Verification items for this drawing (mm, ordinates from the low corner). A direction names the side the tool comes from. Round coordinates to 2 decimals unless told otherwise and drop trailing zeros. Loops run counter-clockwise (first coordinate to the right, second up) from the corner with the lowest first, then second, coordinate; pieces in that order, holes last. Notation, with made-up numbers: M 44,89 L 82,89 A9 cw 82,102 Z; hole C 53,-5 d9. An arc over 180 degrees is marked long. Answer as CSV lines item,"result".
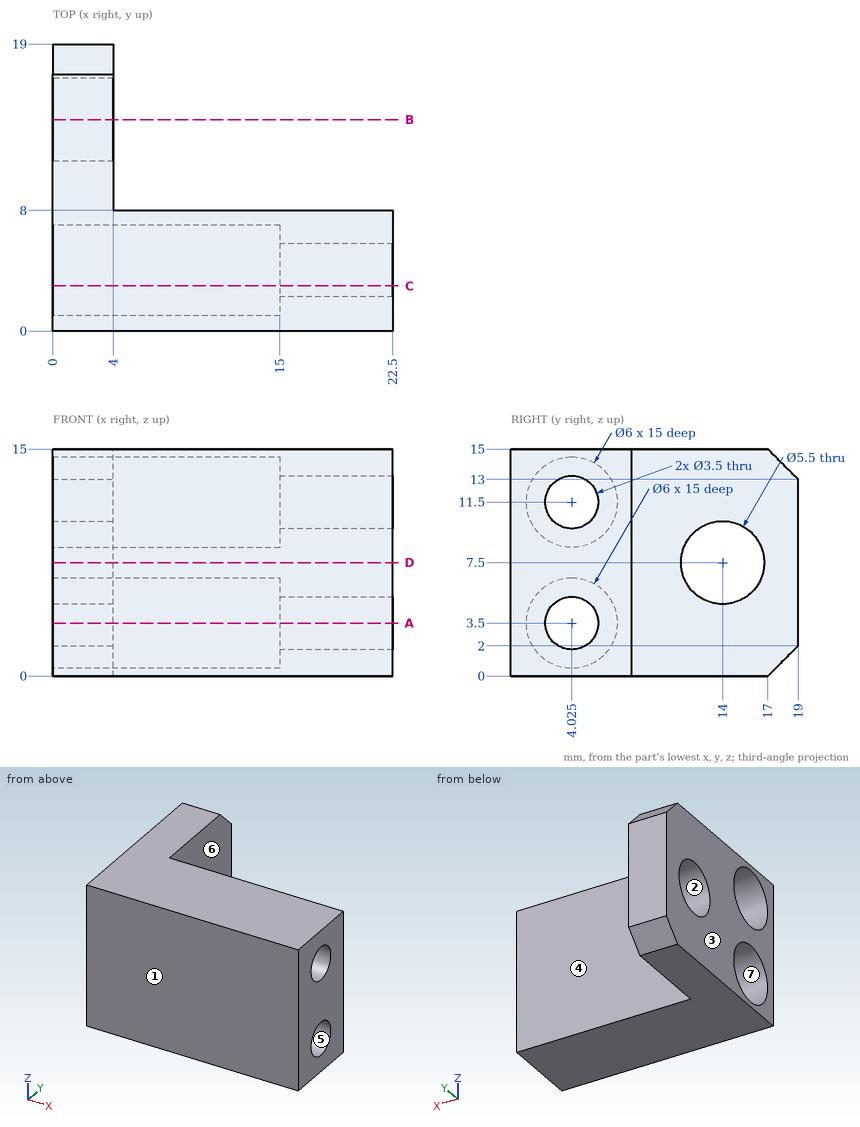
1) Section check C-C (y = 3). Record the cut outline in (x, z).
Here are the results:
outline,"M 0,0 L 22.5,0 L 22.5,2.08 L 15,2.08 L 15,0.68 L 0,0.68 Z; M 0,6.32 L 15,6.32 L 15,4.92 L 22.5,4.92 L 22.5,10.08 L 15,10.08 L 15,8.68 L 0,8.68 Z; M 0,14.32 L 15,14.32 L 15,12.92 L 22.5,12.92 L 22.5,15 L 0,15 Z"
2) Section check B-B (y = 14). Record the cut outline in (x, z), plus the area to 3 significant figures.
Here are the results:
outline,"M 0,0 L 4,0 L 4,4.75 L 0,4.75 Z; M 0,10.25 L 4,10.25 L 4,15 L 0,15 Z"
area,"38.0 mm^2"
3) Draft check along Y on the marked faces 1, 2, 3 and 4. Enter one of: +Y half, -Y half, draft (parallel to the pull), parting line (faces both ways), or undercut.
Here are the results:
face 1,"-Y half"
face 2,"undercut"
face 3,"draft"
face 4,"+Y half"
4) Section check D-D (z = 7.5). Record the cut outline in (x, y).
Here are the results:
outline,"M 0,0 L 22.5,0 L 22.5,8 L 4,8 L 4,11.25 L 0,11.25 Z; M 0,16.75 L 4,16.75 L 4,19 L 0,19 Z"
5) Section check A-A (z = 3.5). Record the cut outline in (x, y) (3 decimals), plus the area to 3 significant figures.
Here are the results:
outline,"M 0,0 L 22.5,0 L 22.5,2.275 L 15,2.275 L 15,1.025 L 0,1.025 Z; M 0,7.025 L 15,7.025 L 15,5.775 L 22.5,5.775 L 22.5,8 L 4,8 L 4,19 L 0,19 Z"
area,"108 mm^2"
6) Material ranges on probe 1 along Y at (x, z) = (2.95, 7.5); probe 2 along Z at (x, y) = (5.25, 3.5); probe 3 along Y at (x, z) = (20.25, 3.5) (3 decimals), recorded low to high.
Here are the results:
probe 1,"y = 0 to 11.25, 16.75 to 19"
probe 2,"z = 0 to 0.55, 6.45 to 8.55, 14.45 to 15"
probe 3,"y = 0 to 2.275, 5.775 to 8"
7) Go/stop test with flat-tipped pins: pin 1 (3 mm diameter, centred on y = 3.5, z = 11, fed in from -X); pin 2 (7 mm diameter, centred on y = 14, z = 7.5, fed in from +X); pin 3 (3 mm diameter, centred on y = 4.03, z = 11.5, fed in from -X); pin 4 (4 mm diameter, centred on x = 12, z = 4.5, fed in from +Y). Record where each tip stops, or that it passes through.
Here are the results:
pin 1,"stops at x = 15"
pin 2,"stops at x = 4"
pin 3,"passes through"
pin 4,"stops at y = 8"
8) Set-up check for the marked faces 5, 6 and 7: record each of +Z, -Z, +X, -X, +Y, -Y from which the full face is reachable in a straight line by a thin tool's end or side.
Here are the results:
face 5,"+X, -X"
face 6,"+Z, -Z, +X, +Y"
face 7,"-X"
